For this review, take the finished solid that the model builds, in its own axes (mm). A direction names the side the tool comes from. Round coordinates to 2 decimals unless told otherwise and drop trailing zeros. Order: outer loops, then holes, each group sorted by start corner. A loop starts at its lowest first (then second) coordinate and runs counter-clockwise, first axis right, second up. Notation, with made-up numbers: (77.5, 78.5) - (99.5, 78.5) arc R25 ccw to (99.5, 117.5) - close; hole circle Ø4 at (-32, -10). An arc over 180 degrees is marked (long way). Write each question's results on one line, items separated by ' | '. Start each with the question number.
(1) Take a section at C-C, the plane x = 14.75. Give the boundary of the cut face in (y, z).
(2) For faces 5 (the cylindrical face through (6.215, -0.949, 0.74)), 6 (the flat face through (0, 3, 1.5)), list the 3-axis set-ups (+Z, -Z, +X, -X, +Y, -Y) from which the entire face can be reached by the end or side of a thin tool; tool diameter is ignored.
(3) Take a section at D-D, the plane z = 0.6. Give the number of separate pieces and of enclosed holes in the cut face, plus the area to 3 significant figures.
(4) Take a section at B-B, the plane y = -0.75. Give the boundary of the cut face in (x, z).
(5) Draft analysis for pull direction Y (two halves, no side actions). For faces 1 (the flat face through (0, -8.75, 1)), 2 (the flat face through (0, -12.5, 1)), 3 (the cylindrical face through (19.465, 12.199, 0.74)), 4 (the flat face through (0, 8.75, 1)), state which applies: pulls with the +Y half, pulls with the -Y half, needs draft (parallel to the pull), parting line crosses it, or undercut.
(6) Take a section at A-A, the plane x = -3.5. Give the boundary of the cut face in (y, z).
(7) For L1, parallel to Y at x = -3, z = 0.5; L2, parallel to Y at x = -14.75, z = 1.15; L3, parallel to X at y = 0, z = 0.3, list the stretches that pass through material, from the lowest coordinate up. Write a range as from..to.
```python
from build123d import *

# Parameters (mm, degrees)
F0_R     = 1.1
F1_DEPTH = 1.5


with BuildPart() as f1:
    # F0 (on Top) → F1 (new body)
    with BuildSketch(Plane.XY):
        with BuildLine():
            ThreePointArc((19.75, 11.5), (19.457107, 12.207107), (18.75, 12.5))
            Line((18.75, 12.5), (-18.75, 12.5))
            ThreePointArc((-18.75, 12.5), (-19.457107, 12.207107), (-19.75, 11.5))
            Line((-19.75, 11.5), (-19.75, -11.5))
            ThreePointArc((-19.75, -11.5), (-19.457107, -12.207107), (-18.75, -12.5))
            Line((-18.75, -12.5), (18.75, -12.5))
            ThreePointArc((18.75, -12.5), (19.457107, -12.207107), (19.75, -11.5))
            Line((19.75, -11.5), (19.75, 11.5))
        make_face()
        with Locations((-14.75, -7.5)):
            Circle(F0_R, mode=Mode.SUBTRACT)
        with BuildLine():
            ThreePointArc((-5.5, -8.75), (-6.207107, -8.457107), (-6.5, -7.75))
            Line((-6.5, -7.75), (-6.5, -7.25))
            ThreePointArc((-6.5, -7.25), (-6.207107, -6.542893), (-5.5, -6.25))
            Line((-5.5, -6.25), (5.5, -6.25))
            ThreePointArc((5.5, -6.25), (6.207107, -6.542893), (6.5, -7.25))
            Line((6.5, -7.25), (6.5, -7.75))
            ThreePointArc((6.5, -7.75), (6.207107, -8.457107), (5.5, -8.75))
            Line((5.5, -8.75), (-5.5, -8.75))
        make_face(mode=Mode.SUBTRACT)
        with Locations((14.75, -7.5)):
            Circle(F0_R, mode=Mode.SUBTRACT)
        with Locations((-14.75, 7.5)):
            Circle(F0_R, mode=Mode.SUBTRACT)
        with BuildLine():
            ThreePointArc((-6.5, 0.25), (-6.207107, 0.957107), (-5.5, 1.25))
            Line((-5.5, 1.25), (5.5, 1.25))
            ThreePointArc((5.5, 1.25), (6.207107, 0.957107), (6.5, 0.25))
            Line((6.5, 0.25), (6.5, -0.25))
            ThreePointArc((6.5, -0.25), (6.207107, -0.957107), (5.5, -1.25))
            Line((5.5, -1.25), (-5.5, -1.25))
            ThreePointArc((-5.5, -1.25), (-6.207107, -0.957107), (-6.5, -0.25))
            Line((-6.5, -0.25), (-6.5, 0.25))
        make_face(mode=Mode.SUBTRACT)
        with BuildLine():
            ThreePointArc((-6.5, 7.75), (-6.207107, 8.457107), (-5.5, 8.75))
            Line((-5.5, 8.75), (5.5, 8.75))
            ThreePointArc((5.5, 8.75), (6.207107, 8.457107), (6.5, 7.75))
            Line((6.5, 7.75), (6.5, 7.25))
            ThreePointArc((6.5, 7.25), (6.207107, 6.542893), (5.5, 6.25))
            Line((5.5, 6.25), (-5.5, 6.25))
            ThreePointArc((-5.5, 6.25), (-6.207107, 6.542893), (-6.5, 7.25))
            Line((-6.5, 7.25), (-6.5, 7.75))
        make_face(mode=Mode.SUBTRACT)
        with Locations((14.75, 7.5)):
            Circle(F0_R, mode=Mode.SUBTRACT)
    extrude(amount=F1_DEPTH)


solid = f1.part
```
Results below:
1) outline: (-12.5, 0) - (-8.6, 0) - (-8.6, 1.5) - (-12.5, 1.5) - close; (-6.4, 0) - (6.4, 0) - (6.4, 1.5) - (-6.4, 1.5) - close; (8.6, 0) - (12.5, 0) - (12.5, 1.5) - (8.6, 1.5) - close
2) face 5: +Z, -Z | face 6: +Z, +X, -X, +Y, -Y
3) separate pieces: 1 | enclosed holes: 7 | area: 877 mm^2
4) outline: (-19.75, 0) - (-6.37, 0) - (-6.37, 1.5) - (-19.75, 1.5) - close; (6.37, 0) - (19.75, 0) - (19.75, 1.5) - (6.37, 1.5) - close
5) face 1: undercut | face 2: pulls with the -Y half | face 3: pulls with the +Y half | face 4: undercut
6) outline: (-12.5, 0) - (-8.75, 0) - (-8.75, 1.5) - (-12.5, 1.5) - close; (-6.25, 0) - (-1.25, 0) - (-1.25, 1.5) - (-6.25, 1.5) - close; (1.25, 0) - (6.25, 0) - (6.25, 1.5) - (1.25, 1.5) - close; (8.75, 0) - (12.5, 0) - (12.5, 1.5) - (8.75, 1.5) - close
7) L1: y = -12.5..-8.75, -6.25..-1.25, 1.25..6.25, 8.75..12.5 | L2: y = -12.5..-8.6, -6.4..6.4, 8.6..12.5 | L3: x = -19.75..-6.5, 6.5..19.75
